Can you work these out from the drawing? Everything is in mm from the part's minimum corner. A direction names the side the tool comes from. Round coordinates to 2 decimals unless told otherwise and drop trailing zeros. Write each loop counter-clockwise with the first axis right and the second up, starting at its lowest first coordinate (ties: lowest second). Pieces come first, ordered by that corner, then holes.
Q1. If we section it at D-D (z = 0.75): Please give me the cut outline in (x, y), plus the area to 3 significant figures.
Q2. We'd pull the mould along Z, two halves only. Please class the marked faces 1, 2 and 3: +Z half, -Z half, draft (parallel to the pull), parting line (faces both ways), or undercut.
Q3. If we section it at C-C (x = 0.9): Please give me the cut outline in (y, z).
Q4. If we section it at A-A (z = 5): Please give me the cut outline in (x, y).
Q5. Please list where these lines run through material, in increasing order: line 1 along Y through (x, z) = (1.1, 3.5); line 2 along Y through (x, z) = (1.45, 5).
Q6. For the marked faces 4, 5 and 6, which set-ups out of +Z, -Z, +X, -X, +Y, -Y let a thin tool reach every point of the face, with its end or its side?
Q7. If we section it at B-B (y = 6.5): Please give me the cut outline in (x, z), plus the area to 3 significant figures.
Q8. I'm going to push flat-ended pins straight in: pin 1 Ø2 at (y, z) = (2.5, 5.5) entering from -X; pin 2 Ø1.1 at (x, z) = (3, 3) entering from +Y; pin 3 Ø2 at (x, y) = (3.5, 1) entering from -Z. Where does each tip first touch, or does it pass through?
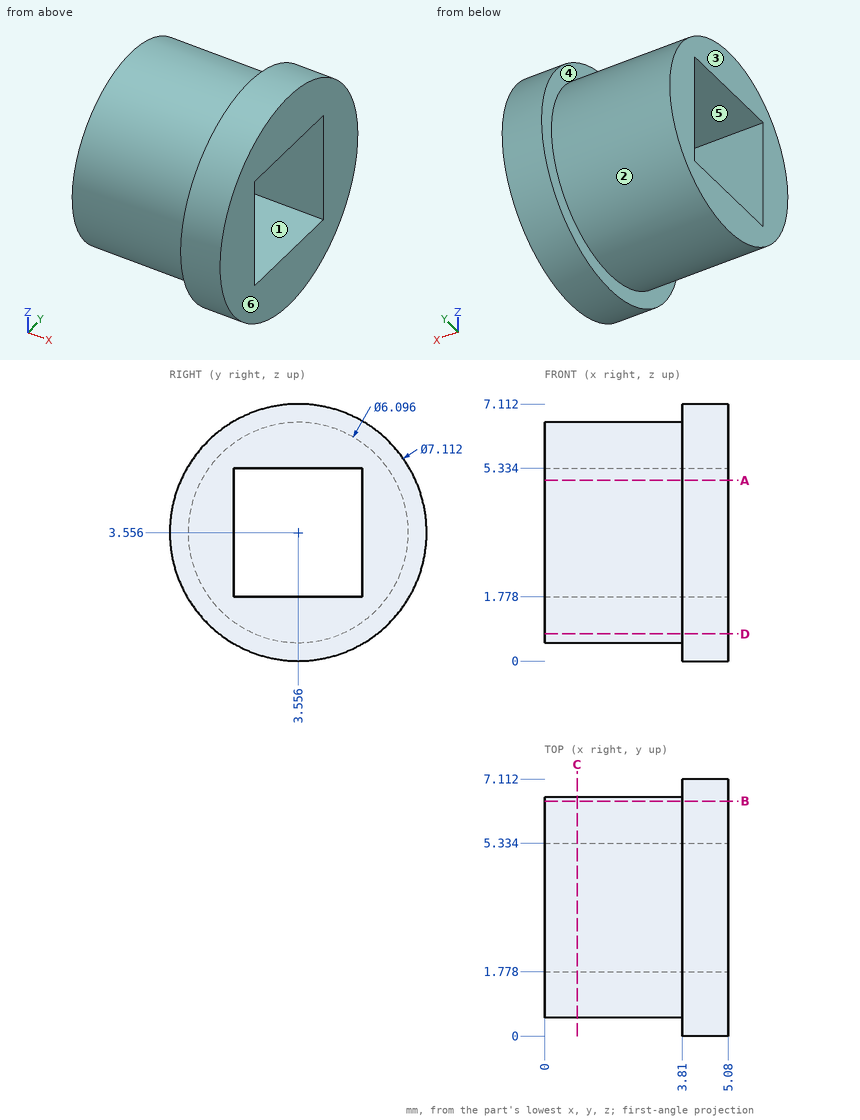
A:
1. outline: (0, 2.37) - (3.81, 2.37) - (3.81, 1.37) - (5.08, 1.37) - (5.08, 5.74) - (3.81, 5.74) - (3.81, 4.75) - (0, 4.75) - close
1. area: 14.6 mm2
2. face 1: undercut
2. face 2: parting line
2. face 3: draft
3. outline: circle Ø6.1 at (3.56, 3.56); hole (1.78, 1.78) - (5.33, 1.78) - (5.33, 5.33) - (1.78, 5.33) - close
4. outline: (0, 0.87) - (3.81, 0.87) - (3.81, 0.31) - (5.08, 0.31) - (5.08, 1.78) - (0, 1.78) - close; (0, 5.33) - (5.08, 5.33) - (5.08, 6.81) - (3.81, 6.81) - (3.81, 6.24) - (0, 6.24) - close
5. line 1: y = 0.51 to 1.78, 5.33 to 6.6
5. line 2: y = 0.87 to 1.78, 5.33 to 6.24
6. face 4: -X
6. face 5: +X, -X
6. face 6: +Z, -Z, +X, +Y, -Y
7. outline: (0, 2.77) - (3.81, 2.77) - (3.81, 1.56) - (5.08, 1.56) - (5.08, 5.55) - (3.81, 5.55) - (3.81, 4.35) - (0, 4.35) - close
7. area: 11.1 mm2
8. pin 1: stops at x = 0
8. pin 2: stops at y = 6.6
8. pin 3: stops at z = 0.38
